Here's how the part is built. I have some questions about the finished solid (model axes, mm). A direction names the side the tool comes from. Coordinates: 2 decimals unless noted, no trailing zeros. Order: outer loops, then holes, each group sorted by start corner. A loop starts at its lowest first (then second) coordinate and runs counter-clockwise, first axis right, second up.
```python
from build123d import *

# Parameters (mm, degrees)
MODEL_R                  = 1.8
MODEL_R_2                = 3
RESSALTO_EXTRUS_O1_DEPTH = 6


with BuildPart() as part:
    # Model → Ressalto-extrusão1 (new body)
    with BuildSketch(Plane.XY):
        with BuildLine():
            Line((27.28416807, 8.306820103), (27.28416807, 31.906820103))
            Line((27.28416807, 31.906820103), (82.28416807, 31.906820103))
            Line((82.28416807, 31.906820103), (82.28416807, 8.306820103))
            Line((82.28416807, 8.306820103), (65.88416807, 8.306820103))
            Line((65.88416807, 8.306820103), (65.88416807, 11.806820103))
            ThreePointArc((65.88416807, 11.806820103), (59.88416807, 17.806820103), (53.88416807, 11.806820103))
            Line((53.88416807, 11.806820103), (53.88416807, 8.306820103))
            Line((53.88416807, 8.306820103), (27.28416807, 8.306820103))
        make_face()
        with Locations((78.28416807, 12.806820103)):
            Circle(MODEL_R, mode=Mode.SUBTRACT)
        with Locations((42.86558438, 12.806820103)):
            Circle(MODEL_R_2, mode=Mode.SUBTRACT)
        with Locations((31.28416807, 12.806820103)):
            Circle(MODEL_R, mode=Mode.SUBTRACT)
    extrude(amount=RESSALTO_EXTRUS_O1_DEPTH)


solid = part.part
```
Q1. If we section it at A-A on x = 79.5: Write out the boundary of the cut face in (y, z), then the cut area to 3 significant figures.
Q2. If we section it at D-D on x = 32: Write out the boundary of the cut face in (y, z), then the cut area to 3 significant figures.
Q3. I need wall thicknesses on L1, parallel to Y at x = 32.5, z = 1.2; L2, parallel to X at y = 10.25, z = 3; L3, parallel to Y at x = 42, z = 5.15. Which ranges of each line are inside material? Lowest first, please.
Q4. We'd pull the mould along X, two halves only. Please class faces 3 (the cylindrical face through (60.016, 17.805, 2.958)), 4 (the flat face through (27.284, 20, 3)), 5 (the flat face through (41, 8.307, 3)): pulls with the +X half, pulls with the -X half, needs draft (parallel to the pull), parting line crosses it, or undercut.
Q5. If we section it at C-C on y = 13.75: Write out the boundary of the cut face in (x, z), then the cut area to 3 significant figures.
Q6. For faces 1 (the flat face through (65.884, 10, 3)), 2 (the cylindrical face through (79.95, 12.12, 2.96)), which set-ups out of +Z, -Z, +X, -X, +Y, -Y let a thin tool reach every point of the face, with its end or its side?
Q7. If we section it at B-B on z = 4.1: Write out the boundary of the cut face in (x, y), then the cut area to 3 significant figures.
Reply:
1. outline: (8.31, 0) - (11.48, 0) - (11.48, 6) - (8.31, 6) - close; (14.13, 0) - (31.91, 0) - (31.91, 6) - (14.13, 6) - close
1. area: 126 mm2
2. outline: (8.31, 0) - (11.16, 0) - (11.16, 6) - (8.31, 6) - close; (14.46, 0) - (31.91, 0) - (31.91, 6) - (14.46, 6) - close
2. area: 122 mm2
3. L1: y = 8.31 to 11.48, 14.13 to 31.91
3. L2: x = 27.28 to 41.3, 44.43 to 53.88, 65.88 to 82.28
3. L3: y = 8.31 to 9.93, 15.68 to 31.91
4. face 3: undercut
4. face 4: pulls with the -X half
4. face 5: needs draft
5. outline: (27.28, 0) - (29.75, 0) - (29.75, 6) - (27.28, 6) - close; (32.82, 0) - (40.02, 0) - (40.02, 6) - (32.82, 6) - close; (45.71, 0) - (54.21, 0) - (54.21, 6) - (45.71, 6) - close; (65.56, 0) - (76.75, 0) - (76.75, 6) - (65.56, 6) - close; (79.82, 0) - (82.28, 0) - (82.28, 6) - (79.82, 6) - close
5. area: 191 mm2
6. face 1: +Z, -Z, -Y
6. face 2: +Z, -Z
7. outline: (27.28, 8.31) - (53.88, 8.31) - (53.88, 11.81) arc R6 cw to (65.88, 11.81) - (65.88, 8.31) - (82.28, 8.31) - (82.28, 31.91) - (27.28, 31.91) - close; hole circle Ø3.6 at (31.28, 12.81); hole circle Ø6 at (42.87, 12.81); hole circle Ø3.6 at (78.28, 12.81)
7. area: 1,150 mm2
